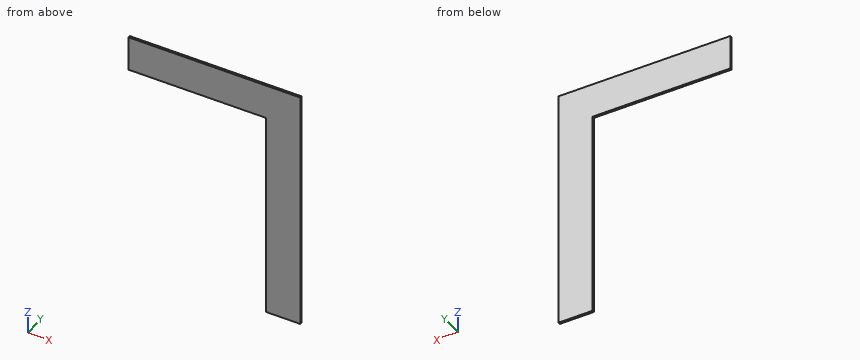
from build123d import *

# Parameters (mm, degrees)
F0_W     = 50.8
F0_H     = 304.8
F1_DEPTH = 3.175


with BuildPart() as f1:
    # F0 (on Front) → F1 (new body)
    with BuildSketch(Plane.XZ):
        with Locations((-25.4, 152.4)):
            Rectangle(F0_W, F0_H)
        Polygon((-50.8, 304.8), (0, 304.8), (0, 355.6), (-254, 355.6), (-254, 304.8), align=None)
    extrude(amount=-F1_DEPTH)


solid = f1.part
Input: part model. Units: mm. Frame: model coordinates. Coordinates: 2 decimals unless noted, no trailing zeros. Order: outer loops, then holes, each group sorted by start corner. A loop starts at its lowest first (then second) coordinate and runs counter-clockwise, first axis right, second up.
1. Contact query for a flat-ended pin moving along its axis: P1, Ø1, axis at y = 2, z = 94.5, coming from the -X side. Output: stop coordinate, or through.
Checked values:
P1: stops at x = -50.8
2. Cut plane B-B, the plane y = 0.5. Return loops of the section in (x, z).
Checked values:
outline: (-254, 304.8) - (-50.8, 304.8) - (-50.8, 0) - (0, 0) - (0, 355.6) - (-254, 355.6) - close
3. Cut plane C-C, the plane z = 181. Return loops of the section in (x, y) (3 decimals).
Checked values:
outline: (-50.8, 0) - (0, 0) - (0, 3.175) - (-50.8, 3.175) - close
4. Cut plane A-A, the plane x = -159. Return loops of the section in (y, z) (3 decimals), plus the area to 3 significant figures.
Checked values:
outline: (0, 304.8) - (3.175, 304.8) - (3.175, 355.6) - (0, 355.6) - close
area: 161 mm2
5. Ray query, line 1 along Z through (x, y) = (-86.5, 2.3); line 2 along X through (y, z) = (0.6, 238). Return the intervals inside material, ascending.
Checked values:
line 1: z = 304.8 to 355.6
line 2: x = -50.8 to 0
